Geometry check sheet. Reference: the model listing, model coordinates, mm. Face numbers are marked on the shaded views. A direction names the side the tool comes from. Round coordinates to 2 decimals unless told otherwise and drop trailing zeros. Write each loop counter-clockwise with the first axis right and the second up, starting at its lowest first coordinate (ties: lowest second). Pieces come first, ordered by that corner, then holes.
Item 1: Cross-section at C-C (z = 36). Enter the section's corners in (x, y).
Item 2: Scan lines: probe 1 along Y at (x, z) = (0, 42); probe 2 along Y at (x, z) = (-2.5, 9.5); probe 3 along X at (y, z) = (1.75, 43). Record each from-to range of solid material in increasing order.
Item 3: Depth check by flat-ended pin: P1, Ø8, axis at x = 1, z = 8, coming from the +Y side; P2, Ø2, axis at y = -1.5, z = 20.5, coming from the +X side; P3, Ø6, axis at y = -1.5, z = 36, coming from the -X side. Enter the tip coordinate at first touch or a pass-through.
Item 4: Cross-section at A-A (x = 0). Enter the section's corners in (y, z).
Item 5: Access from +Z, -Z, +X, -X, +Y, -Y to the whole of each face (thin tool, end or side, straight path). Record for the marked faces 1 and 2.
from build123d import *

# Parameters (mm, degrees)
SKETCH1_R           = 8.5
BOSS_EXTRUDE1_DEPTH = 40
SKETCH2_R           = 11
BOSS_EXTRUDE2_DEPTH = 5
FILLET1_R           = 3


with BuildPart() as part:
    # Sketch1 → Boss-Extrude1 (new body)
    with BuildSketch(Plane.XY):
        Circle(SKETCH1_R)
    extrude(amount=BOSS_EXTRUDE1_DEPTH)

    # Sketch2 → Boss-Extrude2 (add)
    with BuildSketch(Plane.XY.offset(40)):
        Circle(SKETCH2_R)
    extrude(amount=BOSS_EXTRUDE2_DEPTH)

    # Fillet1
    fillet1_edges = [part.edges().sort_by_distance(p)[0] for p in [
        (-11, 0, 45),
    ]]
    fillet(fillet1_edges, radius=FILLET1_R)


solid = part.part
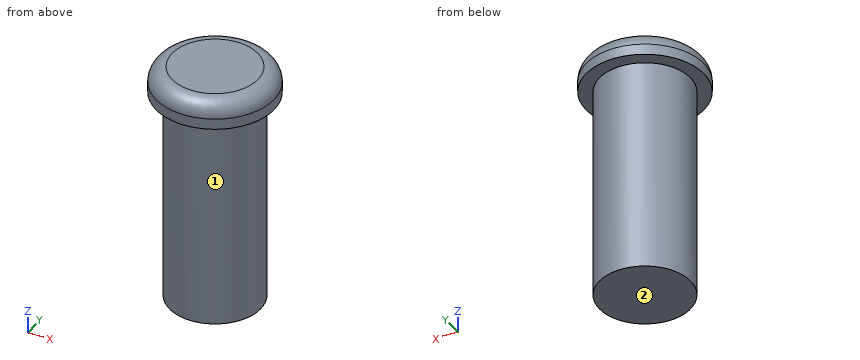
Resolved:
1. outline: circle Ø17 at (0, 0)
2. probe 1: y = -11 to 11
2. probe 2: y = -8.12 to 8.12
2. probe 3: x = -10.69 to 10.69
3. P1: stops at y = 8.5
3. P2: stops at x = 8.49
3. P3: stops at x = -8.5
4. outline: (-11, 40) - (-8.5, 40) - (-8.5, 0) - (8.5, 0) - (8.5, 40) - (11, 40) - (11, 42) arc R3 ccw to (8, 45) - (-8, 45) arc R3 ccw to (-11, 42) - close
5. face 1: -Z
5. face 2: -Z, +X, -X, +Y, -Y
